```python
from build123d import *

# Parameters (mm, degrees)
SKETCH1_R           = 28
BOSS_EXTRUDE1_DEPTH = 8
SKETCH2_R           = 1.5
CUT_EXTRUDE1_DEPTH  = 8
SKETCH3_W           = 2
SKETCH3_H           = 5
SKETCH4_R           = 3
BOSS_EXTRUDE2_DEPTH = 3


with BuildPart() as part:
    # Sketch1 → Boss-Extrude1 (new body)
    with BuildSketch(Plane(origin=(0, 0, 0), x_dir=(1, 0, 0), z_dir=(0, 1, 0))):
        with Locations(Location((0, 0, 0), (0, 0, 270))):
            Circle(SKETCH1_R)
        with BuildLine():
            Line((-2.5, 23.869436525), (-3.5, 9.367496998))
            ThreePointArc((-3.5, 9.367496998), (-5.877852523, 8.090169944), (-7.827459581, 6.223413574))
            Line((-7.827459581, 6.223413574), (-21.928640661, 9.753702823))
            ThreePointArc((-21.928640661, 9.753702823), (-14.106846055, 19.416407865), (-2.5, 23.869436525))
        make_face(mode=Mode.SUBTRACT)
        with BuildLine():
            Line((3.5, 9.367496998), (2.5, 23.869436525))
            ThreePointArc((2.5, 23.869436525), (14.106846055, 19.416407865), (21.928640661, 9.753702823))
            Line((21.928640661, 9.753702823), (7.827459581, 6.223413574))
            ThreePointArc((7.827459581, 6.223413574), (5.877852523, 8.090169944), (3.5, 9.367496998))
        make_face(mode=Mode.SUBTRACT)
        with BuildLine():
            Line((9.990578541, -0.43398204), (23.473725633, 4.998420242))
            ThreePointArc((23.473725633, 4.998420242), (22.825356391, -7.416407865), (16.052645256, -17.841316664))
            Line((16.052645256, -17.841316664), (8.337636066, -5.521215883))
            ThreePointArc((8.337636066, -5.521215883), (9.510565163, -3.090169944), (9.990578541, -0.43398204))
        make_face(mode=Mode.SUBTRACT)
        with BuildLine():
            Line((2.674517106, -9.635712649), (12.007560284, -20.780242925))
            ThreePointArc((12.007560284, -20.780242925), (0, -24), (-12.007560284, -20.780242925))
            Line((-12.007560284, -20.780242925), (-2.674517106, -9.635712649))
            ThreePointArc((-2.674517106, -9.635712649), (0, -10), (2.674517106, -9.635712649))
        make_face(mode=Mode.SUBTRACT)
        with BuildLine():
            Line((-8.337636066, -5.521215883), (-16.052645256, -17.841316664))
            ThreePointArc((-16.052645256, -17.841316664), (-22.825356391, -7.416407865), (-23.473725633, 4.998420242))
            Line((-23.473725633, 4.998420242), (-9.990578541, -0.43398204))
            ThreePointArc((-9.990578541, -0.43398204), (-9.510565163, -3.090169944), (-8.337636066, -5.521215883))
        make_face(mode=Mode.SUBTRACT)
    extrude(amount=BOSS_EXTRUDE1_DEPTH)

    # Sketch2 → Cut-Extrude1 (cut)
    with BuildSketch(Plane(origin=(0, 8, 0), x_dir=(1, 0, 0), z_dir=(0, 1, 0))):
        with Locations(Location((-6.35, 0, 0), (0, 0, 270))):
            Circle(SKETCH2_R)
        with Locations(Location((6.35, 0, 0), (0, 0, 270))):
            Circle(SKETCH2_R)
    extrude(amount=-CUT_EXTRUDE1_DEPTH, mode=Mode.SUBTRACT)

    # Sweep1: sweep along a curve in space
    with BuildLine() as sweep1_path:
        ThreePointArc((0, 8, 28), (19.798989873, 8, 19.798989873), (28, 8, 0))
        ThreePointArc((28, 8, 0), (19.798989873, 8, -19.798989873), (0, 8, -28))
        ThreePointArc((0, 8, -28), (-19.798989873, 8, -19.798989873), (-28, 8, 0))
        ThreePointArc((-28, 8, 0), (-19.798989873, 8, 19.798989873), (0, 8, 28))
    # Sketch3 → Sweep1 (sweep)
    with BuildSketch(Plane(origin=(0, 0, 0), x_dir=(0, 0, -1), z_dir=(1, 0, 0))):
        with Locations((29, 4)):
            Rectangle(SKETCH3_W, SKETCH3_H)
    sweep(path=sweep1_path.line)

    # Sketch4 → Boss-Extrude2 (add)
    with BuildSketch(Plane(origin=(0, 8, 0), x_dir=(1, 0, 0), z_dir=(0, 1, 0))):
        with Locations(Location((0, 0, 0), (0, 0, 270))):
            Circle(SKETCH4_R)
    extrude(amount=BOSS_EXTRUDE2_DEPTH)


solid = part.part
```
The model under review builds one solid part; all positions refer to its coordinate system, in mm. A direction names the side the tool comes from. Round coordinates to 2 decimals unless told otherwise and drop trailing zeros. Loops run counter-clockwise (first coordinate to the right, second up) from the corner with the lowest first, then second, coordinate; pieces in that order, holes last.
Item 1: Take a section at B-B (y = 5). Write out the cut boundary in (x, z), then the cut area to 3 significant figures.
Determined:
outline: circle Ø60 at (0, 0); hole (-23.47, -5) - (-9.99, 0.43) arc R10 cw to (-8.34, 5.52) - (-16.05, 17.84) arc R24 ccw to start; hole (-21.93, -9.75) arc R24 ccw to (-2.5, -23.87) - (-3.5, -9.37) arc R10 cw to (-7.83, -6.22) - close; hole (-12.01, 20.78) - (-2.67, 9.64) arc R10 cw to (2.67, 9.64) - (12.01, 20.78) arc R24 ccw to start; hole circle Ø3 at (-6.35, 0); hole (2.5, -23.87) arc R24 ccw to (21.93, -9.75) - (7.83, -6.22) arc R10 cw to (3.5, -9.37) - close; hole circle Ø3 at (6.35, 0); hole (8.34, 5.52) arc R10 cw to (9.99, 0.43) - (23.47, -5) arc R24 ccw to (16.05, 17.84) - close
area: 1,740 mm2
Item 2: Clearance check with flat-ended pins moving along their axes: pin 1 Ø17 at (x, z) = (14, -13) entering from +Y; pin 2 Ø1 at (y, z) = (5.5, -4) entering from -X; pin 3 Ø3 at (x, y) = (-9.5, 3) entering from -Z; pin 4 Ø1.8 at (x, z) = (6.35, 0) entering from +Y. State where each tip first meets the part, or that it passes through.
Determined:
pin 1: stops at y = 8
pin 2: stops at x = -29.8
pin 3: stops at z = -28.91
pin 4: passes through
Item 3: Take a section at C-C (x = 14). Write out the cut boundary in (y, z).
Determined:
outline: (0, -24.25) - (1.5, -24.25) - (1.5, -26.53) - (6.5, -26.53) - (6.5, -24.25) - (8, -24.25) - (8, -19.49) - (0, -19.49) - close; (0, -7.77) - (8, -7.77) - (8, -1.18) - (0, -1.18) - close; (0, 14.56) - (8, 14.56) - (8, 24.25) - (6.5, 24.25) - (6.5, 26.53) - (1.5, 26.53) - (1.5, 24.25) - (0, 24.25) - close
Item 4: Take a section at D-D (z = 16). Write out the cut boundary in (x, y).
Determined:
outline: (-25.38, 1.5) - (-22.98, 1.5) - (-22.98, 0) - (-17.89, 0) - (-17.89, 8) - (-22.98, 8) - (-22.98, 6.5) - (-25.38, 6.5) - close; (-14.9, 0) - (-8, 0) - (-8, 8) - (-14.9, 8) - close; (8, 0) - (14.9, 0) - (14.9, 8) - (8, 8) - close; (17.89, 0) - (22.98, 0) - (22.98, 1.5) - (25.38, 1.5) - (25.38, 6.5) - (22.98, 6.5) - (22.98, 8) - (17.89, 8) - close
Item 5: For faces 4 (the face through (-16.83, 3.94, -2.32)), 5 (the face through (-27, 1.5, -8)), list the 3-axis set-ups (+Z, -Z, +X, -X, +Y, -Y) from which the entire face can be reached by the end or side of a thin tool; tool diameter is ignored.
Determined:
face 4: +Y, -Y
face 5: -Y
Item 6: For line 1 (Z direction, x = 7, y = 5.25); line 2 (X direction, y = 7.75, z = -18.5); line 3 (X direction, y = 2.25, z = 0), list the stretches that pass through material, from the lowest coordinate up.
Determined:
line 1: z = -29.17 to -22.96, -7.14 to -1.35, 1.35 to 14.8, 22.96 to 29.17
line 2: x = -21.02 to -15.29, -2.87 to 2.87, 15.29 to 21.02
line 3: x = -30 to -24, -11.07 to -7.85, -4.85 to 4.85, 7.85 to 11.07, 24 to 30
Item 7: Mouldability with a two-part tool opening along Z and no side actions: class faces 1 (the face through (16.638, 3.944, -2.244)), 2 (the face through (-8, 6.5, -27)), 3 (the face through (-27.334, 7.24, -6.07)) as released by +Z, released by -Z, zero draft, split by the parting line, or undercut.
Determined:
face 1: undercut
face 2: zero draft
face 3: split by the parting line
Item 8: Take a section at A-A (z = -20.5). Write out the cut boundary in (x, y), then the cut area to 3 significant figures.
Determined:
outline: (-21.9, 1.5) - (-19.07, 1.5) - (-19.07, 0) - (-12.48, 0) - (-12.48, 8) - (-19.07, 8) - (-19.07, 6.5) - (-21.9, 6.5) - close; (-2.73, 0) - (2.73, 0) - (2.73, 8) - (-2.73, 8) - close; (12.48, 0) - (19.07, 0) - (19.07, 1.5) - (21.9, 1.5) - (21.9, 6.5) - (19.07, 6.5) - (19.07, 8) - (12.48, 8) - close
area: 178 mm2
